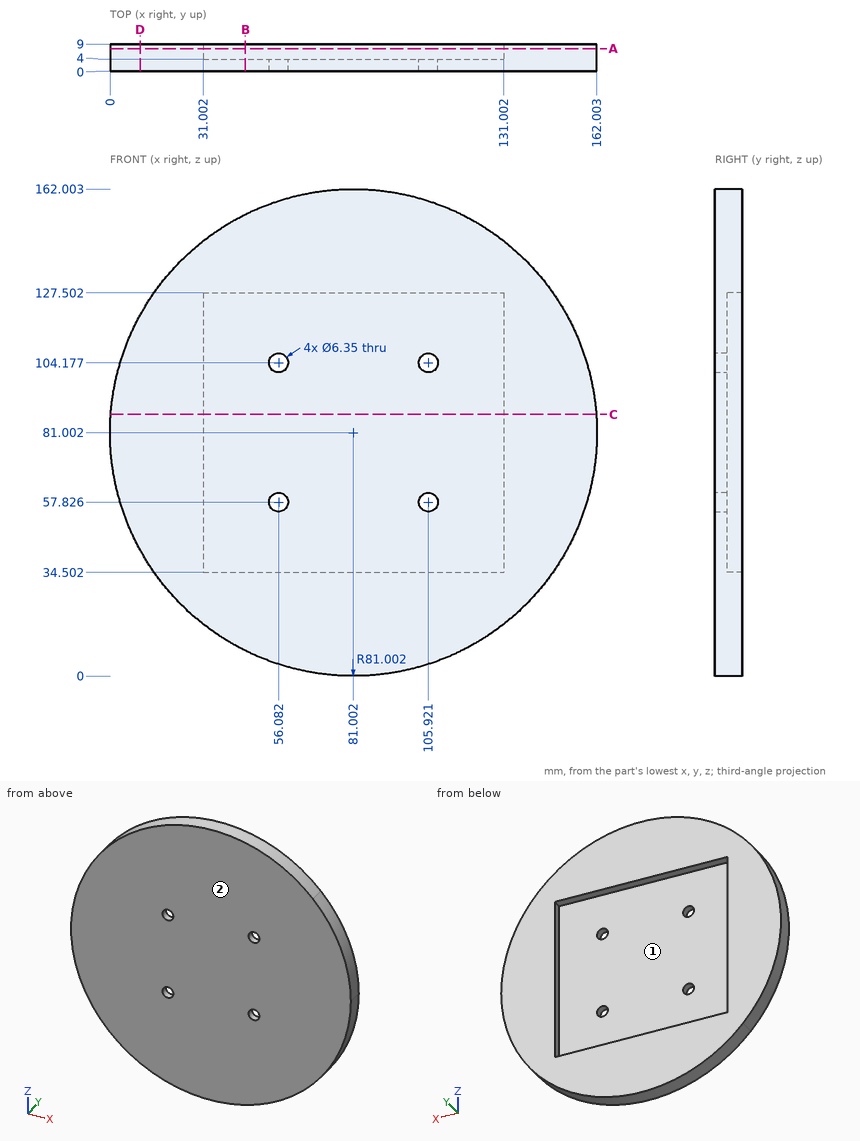
Geometry: see drawing. Coordinates: mm, zero at the bounding-box minimum. Give positions to 0.01 mm unless a question says otherwise; leave off trailing zeros. Loops run counter-clockwise (first coordinate to the right, second up) from the corner with the lowest first, then second, coordinate; pieces in that order, holes last. Notation, with made-up numbers: (42.5, 69) - (68.5, 69) arc R9 ccw to (68.5, 79) - close; hole circle Ø3 at (-1.75, -1). An arc over 180 degrees is marked (long way). Answer as CSV lines item,"result". Start each with the question number.
1. Section B-B, the plane x = 45. Return loops of the section in (y, z), plus the area to 3 significant figures.
2. Section D-D, the plane x = 10. Return loops of the section in (y, z), plus the area to 3 significant figures.
3. Section C-C, the plane z = 87. Return loops of the section in (x, y), plus the area to 3 significant figures.
4. Section A-A, the plane y = 7.5. Return loops of the section in (x, z).
5. Ray query, L1, parallel to Z at x = 107, y = 2 (1 decimal); L2, parallel to X at y = 1, z = 79 (1 decimal); L3, parallel to Z at x = 53, y = 6.5 (1 decimal). Return the intervals inside material, ascending.
6. Draft query along Y for the marked faces 1 and 2. Return one class per face: released by +Y, released by -Y, zero draft, split by the parting line, or undercut.
7. Pin query (flat end, axial travel): P1, Ø4, axis at x = 93.5, y = 7.5, coming from the +Z side; P2, Ø4, axis at y = 7.5, z = 66.5, coming from the -X side; P3, Ø3, axis at x = 57.5, y = 1.5, coming from the +Z side. Return the tip coordinate at first contact, or that it passes through.
Answers:
1,outline,"(0, 8.44) - (9, 8.44) - (9, 34.5) - (4, 34.5) - (4, 127.5) - (9, 127.5) - (9, 153.56) - (0, 153.56) - close"
1,area,"841 mm2"
2,outline,"(0, 42.01) - (9, 42.01) - (9, 119.99) - (0, 119.99) - close"
2,area,"702 mm2"
3,outline,"(0.22, 0) - (161.78, 0) - (161.78, 9) - (131, 9) - (131, 4) - (31, 4) - (31, 9) - (0.22, 9) - close"
3,area,"954 mm2"
4,outline,"circle Ø162 at (81, 81); hole (31, 34.5) - (131, 34.5) - (131, 127.5) - (31, 127.5) - close"
5,L1,"z = 4.3 to 54.8, 60.8 to 101.2, 107.2 to 157.7"
5,L2,"x = 0 to 162"
5,L3,"z = 5 to 34.5, 127.5 to 157"
6,face 1,"released by +Y"
6,face 2,"released by -Y"
7,P1,"stops at z = 161.32"
7,P2,"stops at x = 0.97"
7,P3,"stops at z = 158.96"
